Could you check a few things on this model? Use its own coordinates, in mm. Face numbers are marked on the shaded views. A direction names the side the tool comes from. Give positions to 0.01 mm unless a question says otherwise; leave off trailing zeros. Write each loop counter-clockwise with the first axis right and the second up, starting at its lowest first coordinate (ties: lowest second). Pieces come first, ordered by that corner, then holes. Notation, with made-up numbers: (72, 66) - (101, 66) arc R26 ccw to (101, 85) - close; hole circle Ø11 at (-22.5, -38). An arc over 180 degrees is marked (long way). Write item = value, one per line.
Autodesk Inventor part; units mm, degrees
ref_plane "YZ Plane" through (0, 0, 0) normal (1, 0, 0) x (0, 1, 0)
ref_plane "XZ Plane" through (0, 0, 0) normal (0, 1, 0) x (-1, 0, 0)
ref_plane "XY Plane" through (0, 0, 0) normal (0, 0, 1) x (1, 0, 0)
sketch "Sketch5" plane through (0, 0, 0) normal (0, 0, 1) x (1, 0, 0)
  line L0 (52.8, -15.6) -> (52.8, -10.6)
  line L1 (52.8, -10.6) -> (49.8, -10.6)
  line L2 (49.8, -10.6) -> (49.8, -12.55)
  line L3 (44, -12.55) -> (44, -3.05)
  line L4 (49.8, -3.05) -> (49.8, -5)
  line L5 (49.8, -5) -> (52.8, -5)
  line L6 (52.8, -5) -> (52.8, 0)
  line L7 (52.8, 0) -> (7.8, 0)
  line L8 (44, -3.05) -> (49.8, -3.05)
  line L9 (44, -12.55) -> (49.8, -12.55)
  line L10 (52.8, -15.6) -> (7.8, -15.6)
  arc A0 (7.8, 0) -> (7.8, -15.6) centre (7.8, -7.8) ccw
  point P0 (0, 0)
  dimension "d41" = 5.8
  dimension "d48" = 44
  dimension "d50" = 3
  dimension "d63" = 45
  dimension "d67" = 15.6
  dimension "d71" = 0
  dimension "d72" = 36.2
  dimension "d87" = 5.6
  dimension "d88" = 9.5
extrude "Extrusion2" add sketch "Sketch5" along normal blind 12
sketch "Sketch11" plane through (0, 0, 12) normal (0, 0, 1) x (1, 0, 0)
  line L0 (52.8, 0) -> (7.8, 0)
  line L1 (13.7629, 0) -> (14.8048, -5.9088)
  line L2 (14.8048, -5.9088) -> (0.0327, -8.5136)
  arc A0 (7.8, 0) -> (7.8, -15.6) centre (7.8, -7.8) ccw
  point P0 (0, 0)
  dimension "d95" = 100
  dimension "d96" = 6
  dimension "d97" = 15
extrude "Extrusion7" cut sketch "Sketch11" along normal blind 10 from surface at -12
sketch "Sketch14" plane through (0, 0, 12) normal (0, 0, 1) x (1, 0, 0)
  line L0 (2.7571, 4.8295) -> (7.0478, -19.5045)
  line L1 (7.0478, -19.5045) -> (-13.9668, -23.21)
  line L2 (-13.9668, -23.21) -> (-18.2576, 1.124)
  line L3 (-18.2576, 1.124) -> (2.7571, 4.8295)
  line L4 (13.7629, 0) -> (14.8048, -5.9088)
  point P0 (0, 0)
  dimension "d111" = 10
extrude "Extrusion10" cut sketch "Sketch14" against normal through all
fillet "Fillet2" radius 15 1 edges at (6.3349, -15.4612, 6)
sketch "Sketch15" plane through (13.7629, 0, 10) normal (0, 0, -1) x (-1, 0, 0)
  line L0 (-39.0371, 0) -> (0, 0)
  arc A0 (-5.1829, -15.6) -> (9.5892, -3.2047) centre (-5.1829, -0.6) ccw
  line L1 (0, 0) -> (9.5892, -3.2047)
  line L2 (0, 0) -> (5.9629, 0)
  arc A1 (9.96, -1.102) -> (5.9629, 0) centre (5.9629, -7.8) ccw
  line L3 (9.5892, -3.2047) -> (9.96, -1.102)
  point P0 (13.7629, 0)
extrude "Extrusion11" cut sketch "Sketch15" against normal blind 10
equation "\"l1\" = 8"
properties part number "Finray_test_8_Kerbe_10deg_V4"
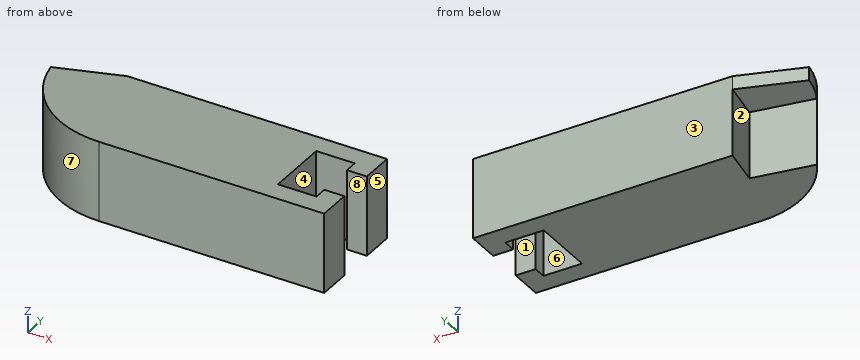
1. If we section it at D-D, the plane y = -13.5: Please give me the cut outline in (x, z), and give its area (3 significant figures).
Filled sheet:
outline = (11.29, 0) - (52.8, 0) - (52.8, 12) - (11.29, 12) - close
area = 498 mm2
2. If we section it at A-A, the plane x = 47.5: Please give me the cut outline in (y, z).
Filled sheet:
outline = (-15.6, 0) - (-12.55, 0) - (-12.55, 12) - (-15.6, 12) - close; (-3.05, 0) - (0, 0) - (0, 12) - (-3.05, 12) - close
3. Thinking about a two-plate mould opening in X: for the marked faces 6, 7 and 8, which applies, pulls with the +X half, pulls with the -X half, needs draft (parallel to the pull), parting line crosses it, or undercut?
Filled sheet:
face_6 = undercut
face_7 = pulls with the -X half
face_8 = needs draft
4. For pin 1 (1.6 mm diameter, centred on y = -3.5, z = 7, fed in from -X); pin 2 (2 mm diameter, centred on y = -11.5, z = 6, fed in from -X), each with a flat end and sliding along its axis, tell me the tip position at first contact or that it passes through.
Filled sheet:
pin_1 = 14.24
pin_2 = 7.68
5. If we section it at B-B, the plane z = 3.5: Please give me the cut outline in (x, y), and give its area (3 significant figures).
Filled sheet:
outline = (5.64, -7.52) arc R15 ccw to (18.95, -15.6) - (52.8, -15.6) - (52.8, -10.6) - (49.8, -10.6) - (49.8, -12.55) - (44, -12.55) - (44, -3.05) - (49.8, -3.05) - (49.8, -5) - (52.8, -5) - (52.8, 0) - (13.76, 0) - (14.8, -5.91) - close
area = 575 mm2
6. If we section it at C-C, the plane y = -10: Please give me the cut outline in (x, z).
Filled sheet:
outline = (7.26, 0) - (44, 0) - (44, 12) - (7.26, 12) - close
7. I need wall thicknesses on line 1 (X direction, y = -10.75, z = 3); line 2 (X direction, y = -11.25, z = 3.75); line 3 (X direction, y = -5.5, z = 1.75). Which ranges of each line are inside material? Lowest first, please.
Filled sheet:
line_1 = 7.9 to 44, 49.8 to 52.8
line_2 = 8.38 to 44, 49.8 to 52.8
line_3 = 14.73 to 44
8. Which directions (+Z, -Z, +X, -X, +Y, -Y) give clear straight access to the entire face, cutting with the end or side of a thin tool? Please do the marked faces 1, 2, 3, 4 and 5.
Filled sheet:
face_1 = +Z, -Z, +X
face_2 = -Z, -X
face_3 = +Z, -Z, +X, -X, +Y
face_4 = +Z, -Z
face_5 = +Z, -Z, +X, +Y, -Y
